Solid Edge part; units mm, degrees
sketch "Sketch1" plane through (0, 0, 0) normal (0, 0, 1) x (1, 0, 0)
  line L0 (-110, -110) -> (110, -110)
  line L1 (110, -110) -> (110, 110)
  line L2 (110, 110) -> (-110, 110)
  line L3 (-110, 110) -> (-110, -110)
extrude "Protrusion1" add sketch "Sketch1" along normal mid plane 10
sketch "Sketch2" plane through (0, 0, -5) normal (0, 0, -1) x (1, 0, 0)
  line L0 (-30, -27.5) -> (30, -27.5)
  line L1 (30, -27.5) -> (30, 27.5)
  line L2 (30, 27.5) -> (-30, 27.5)
  line L3 (-30, 27.5) -> (-30, -27.5)
extrude "ExtrudedCutout_1" cut sketch "Sketch2" against normal blind 3
Read the model definition and answer for the solid it produces. Units are mm, in the model's axes. Round coordinates to 2 decimals unless told otherwise and drop trailing zeros. Write each loop counter-clockwise with the first axis right and the second up, starting at its lowest first coordinate (ties: lowest second). Pieces come first, ordered by that corner, then holes.
1. Straight lines are drawn through the part: L1, parallel to X at y = -11, z = -3.25; L2, parallel to Z at x = 15.5, y = -7.5. For each, find the intervals that lie inside material, in ascending order.
2. Given pin 1 Ø10 at (x, y) = (-22.5, 3) entering from -Z, flat-ended and moving along its own axis, determine where the tip first touches the part or whether it passes through.
3. The part is cut by section A-A, the plane y = -8. Determine the outline of the cut face in (x, z).
4. Determine the mould class of faces 1 (the face through (0, 0, -2)), 2 (the face through (2, 110, 0)), 3 (the face through (-110, 2, 0)), 4 (the face through (110, -2, 0)) for opening direction X: pulls with the +X half, pulls with the -X half, needs draft (parallel to the pull), parting line crosses it, or undercut.
5. The part is cut by section B-B, the plane x = 21. Determine the outline of the cut face in (y, z), then the cut area to 4 significant figures.
Values:
1. L1: x = -110 to -30, 30 to 110
1. L2: z = -2 to 5
2. pin 1: stops at z = -2
3. outline: (-110, -5) - (-30, -5) - (-30, -2) - (30, -2) - (30, -5) - (110, -5) - (110, 5) - (-110, 5) - close
4. face 1: undercut
4. face 2: needs draft
4. face 3: pulls with the -X half
4. face 4: pulls with the +X half
5. outline: (-110, -5) - (-27.5, -5) - (-27.5, -2) - (27.5, -2) - (27.5, -5) - (110, -5) - (110, 5) - (-110, 5) - close
5. area: 2,035 mm2
